```python
from build123d import *

# Parameters (mm, degrees)
SKETCH3_R          = 3.175
CUT_EXTRUDE1_DEPTH = 24.850898387


with BuildPart() as part:
    # Sketch2 → Barbfitting(Mcmaster) (revolve)
    with BuildSketch(Plane(origin=(0, 0, 0), x_dir=(0, 0, -1), z_dir=(1, 0, 0))):
        Polygon((-15.111710887, 0), (-15.111710887, 4.234813167), (-10.754464436, 4.753622494), (-10.754464436, 4.205934994), (-10.605348064, 4.223690006), (-6.154683186, 4.753622494), (-6.154683186, 4.205934994), (-6.005566814, 4.223690006), (-1.554901936, 4.753622494), (-1.554901936, 4.205934994), (-1.405785564, 4.223690006), (3.044879314, 4.753622494), (3.044879314, 4.205934994), (3.193995686, 4.223690006), (7.707996691, 4.76116381), (8.7391875, 4.7625), (8.7391875, 0), align=None)
    revolve(axis=Axis((0, 0, 15.2796875), (0, 0, -1)))

    # Sketch3 → Cut-Extrude1 (cut, through all)
    with BuildSketch(Plane.XY.offset(15.111710887)):
        Circle(SKETCH3_R)
    extrude(amount=-CUT_EXTRUDE1_DEPTH, mode=Mode.SUBTRACT)


solid = part.part
```
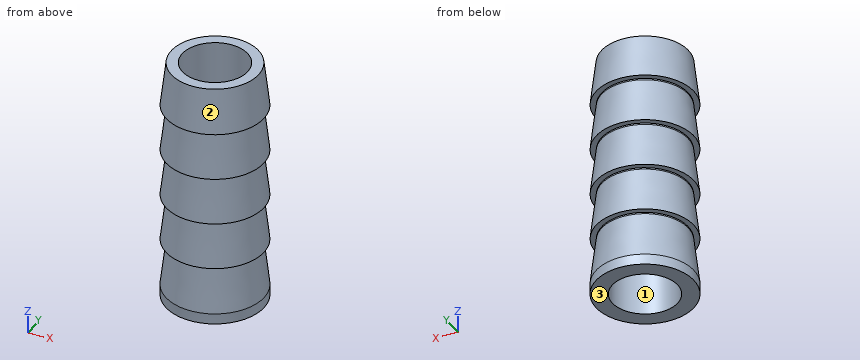
Verification items for the finished model (mm, model axes). Face numbers are marked on the shaded views. Give positions to 0.01 mm unless a question says otherwise; leave off trailing zeros. Loops run counter-clockwise (first coordinate to the right, second up) from the corner with the lowest first, then second, coordinate; pieces in that order, holes last.
1. Mould release check, pull along Y, two halves, no side actions. Record for the marked faces 1, 2 and 3: released by +Y, released by -Y, zero draft, split by the parting line, or undercut.
2. Go/stop test with flat-tipped pins: pin 1 Ø5.5 at (x, y) = (0, 0) entering from -Z; pin 2 Ø3 at (y, z) = (3.5, 1) entering from -X; pin 3 Ø1.5 at (x, y) = (0, -2.5) entering from +Z; pin 4 Ø1.5 at (y, z) = (0, -3) entering from +X. Record where each tip stops, or that it passes through.
3. Section check A-A, the plane z = 5.25. Enter the section's corners in (x, y) (3 decimals), then the cut area to 3 significant figures.
4. Thickness scan on line 1 (X direction, y = -1.5, z = -0.5); line 2 (X direction, y = -2.25, z = 5.25); line 3 (Y direction, x = 0, z = -2.75) (3 decimals). Record the ranges inside material, lowest first.
5. Section check B-B, the plane z = 12. Enter the section's corners in (x, y) (3 decimals), then the cut area to 3 significant figures.
Geometry says:
1. face 1: undercut
1. face 2: split by the parting line
1. face 3: zero draft
2. pin 1: passes through
2. pin 2: stops at x = -4.26
2. pin 3: stops at z = 15.11
2. pin 4: stops at x = 4.75
3. outline: circle Ø8.627 at (0, 0); hole circle Ø6.35 at (0, 0)
3. area: 26.8 mm2
4. line 1: x = -4.19 to -2.8, 2.8 to 4.19
4. line 2: x = -3.68 to -2.24, 2.24 to 3.68
4. line 3: y = -4.719 to -3.175, 3.175 to 4.719
5. outline: circle Ø9.211 at (0, 0); hole circle Ø6.35 at (0, 0)
5. area: 35.0 mm2
